Verification items for the finished model (mm, model axes). Face numbers are marked on the shaded views. A direction names the side the tool comes from. Round coordinates to 2 decimals unless told otherwise and drop trailing zeros. Loops run counter-clockwise (first coordinate to the right, second up) from the corner with the lowest first, then second, coordinate; pieces in that order, holes last. Notation, with made-up numbers: (44, 2) -> (102, 2) arc R17 ccw to (102, 28) -> close; hole circle Ø10 at (6, 40). An arc over 180 degrees is marked (long way). Write item = value, one per line.
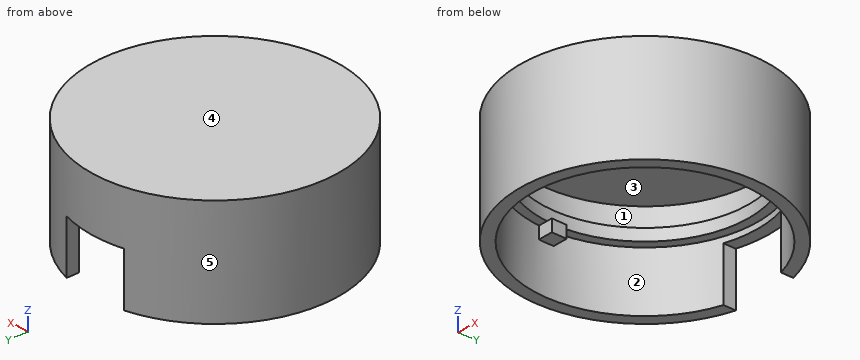
```python
from build123d import *

# Parameters (mm, degrees)
SKIZZE2_W                       = 11
SKIZZE2_H                       = 9
SCHNITT_LINEAR_AUSTRAGEN2_DEPTH = 25
SKIZZE3_W                       = 2.03
SKIZZE3_H                       = 2.5
AUFSATZ_LINEAR_AUSTRAGEN1_DEPTH = 18.902
SKIZZE3_3_W                     = 2.03
SKIZZE3_3_H                     = 2.5
SCHNITT_LINEAR_AUSTRAGEN3_DEPTH = 16.402


with BuildPart() as part:
    # Skizze1 → Rotation2 (revolve)
    with BuildSketch(Plane(origin=(0, 0, 0), x_dir=(1, 0, 0), z_dir=(0, 1, 0)), mode=Mode.PRIVATE) as rotation2_sk:
        Polygon((0.00340061, -8.034840547), (0.00340061, -10.034840547), (20.90540061, -10.034840547), (20.90540061, 7.965159453), (18.90540061, 7.965159453), (18.90540061, -2.034840547), (17.40540061, -2.034840547), (17.40540061, -4.034840547), (18.90540061, -4.034840547), (18.90540061, -8.034840547), align=None)
    revolve(rotation2_sk.sketch.rotate(Axis((0.00340061, 0, 8.034840547), (0, 0, 1)), 180), axis=Axis((0.00340061, 0, 8.034840547), (0, 0, 1)))

    # Skizze2 → Schnitt-Linear austragen2 (cut)
    with BuildSketch(Plane(origin=(0, 0, 0), x_dir=(1, 0, 0), z_dir=(0, 1, 0))):
        with Locations((0.00340061, 3.465159453)):
            Rectangle(SKIZZE2_W, SKIZZE2_H)
    extrude(amount=SCHNITT_LINEAR_AUSTRAGEN2_DEPTH, mode=Mode.SUBTRACT)

    # Skizze3 → Aufsatz-Linear austragen1 (add)
    with BuildSketch(Plane(origin=(0, 0, 0), x_dir=(0, 0, -1), z_dir=(1, 0, 0))):
        with Locations((-1.015, 0)):
            Rectangle(SKIZZE3_W, SKIZZE3_H)
    extrude(amount=-AUFSATZ_LINEAR_AUSTRAGEN1_DEPTH)

    # Skizze3_3 → Schnitt-Linear austragen3 (cut)
    with BuildSketch(Plane(origin=(0, 0, 0), x_dir=(0, 0, -1), z_dir=(1, 0, 0))):
        with Locations((-1.015, 0)):
            Rectangle(SKIZZE3_3_W, SKIZZE3_3_H)
    extrude(amount=-SCHNITT_LINEAR_AUSTRAGEN3_DEPTH, mode=Mode.SUBTRACT)


solid = part.part
```
(1) Sectioned sample at A-A, the plane x = 7.5. Record the cut outline in (y, z), and give its area (3 significant figures).
Filled sheet:
outline = (-19.51, -7.97) -> (-17.35, -7.97) -> (-17.35, 2.03) -> (-15.7, 2.03) -> (-15.7, 4.03) -> (-17.35, 4.03) -> (-17.35, 8.03) -> (17.35, 8.03) -> (17.35, 4.03) -> (15.7, 4.03) -> (15.7, 2.03) -> (17.35, 2.03) -> (17.35, -7.97) -> (19.51, -7.97) -> (19.51, 10.03) -> (-19.51, 10.03) -> close
area = 154 mm2
(2) Go/stop test with flat-tipped pins: pin 1 Ø1.5 at (x, y) = (7.5, -9) entering from -Z; pin 2 Ø3 at (x, y) = (2.5, 20) entering from -Z; pin 3 Ø0.6 at (x, z) = (-17.5, 1.5) entering from -Y. Record where each tip stops, or that it passes through.
Filled sheet:
pin_1 = 8.03
pin_2 = 1.03
pin_3 = -11.87
(3) Sectioned sample at D-D, the plane x = 13. Record the cut outline in (y, z), and give its area (3 significant figures).
Filled sheet:
outline = (-16.37, -7.97) -> (-13.72, -7.97) -> (-13.72, 2.03) -> (-11.57, 2.03) -> (-11.57, 4.03) -> (-13.72, 4.03) -> (-13.72, 8.03) -> (13.72, 8.03) -> (13.72, 4.03) -> (11.57, 4.03) -> (11.57, 2.03) -> (13.72, 2.03) -> (13.72, -7.97) -> (16.37, -7.97) -> (16.37, 10.03) -> (-16.37, 10.03) -> close
area = 159 mm2
(4) Set-up check for the marked faces 1 and 2: record each of +Z, -Z, +X, -X, +Y, -Y from which the full face is reachable in a straight line by a thin tool's end or side.
Filled sheet:
face_1 = none
face_2 = -Z
(5) Draft check along X on the marked faces 3, 4 and 5. Enter one of: released by +X, released by -X, zero draft, split by the parting line, or undercut.
Filled sheet:
face_3 = undercut
face_4 = zero draft
face_5 = split by the parting line
(6) Sectioned sample at C-C, the plane z = 9. Record the cut outline in (x, y), and give its area (3 significant figures).
Filled sheet:
outline = circle Ø41.8 at (0, 0)
area = 1,370 mm2
(7) Material ranges on probe 1 along Z at (x, y) = (12, -13.5); probe 2 along Y at (x, z) = (-17, 0.5); probe 3 along X at (y, z) = (0.5, 3.5), recorded low to high. Write a range as from..to.
Filled sheet:
probe_1 = 2.03..4.03, 8.03..10.03
probe_2 = -12.16..-8.26, -1.25..1.25, 8.26..12.16
probe_3 = -20.89..-17.39, 17.4..20.9
